```python
from build123d import *

# Parameters (mm, degrees)
SKETCH019_R          = 1.7
PAD002_DEPTH         = 13
SKETCH020_W          = 7
SKETCH020_H          = 8
POCKET017_DEPTH      = 7
POCKET019_DEPTH      = 8
POCKET020_DEPTH      = 8
SKETCH024_R          = 2.5
SKETCH025_R          = 10
SKETCH027_R          = 10
SKETCH026_R          = 2.5
SKETCH021_R          = 1.7
POCKET021_DEPTH      = 21.5010001
POCKET021_DEPTH_BACK = 21.5010001
SKETCH028_W          = 57.890867
SKETCH028_H          = 28.005435
SKETCH028_W_2        = 40
SKETCH028_H_2        = 13
POCKET022_DEPTH      = 21.5010001
POCKET022_DEPTH_BACK = 21.5010001
SKETCH029_W          = 10.751613
SKETCH029_H          = 15.361299
POCKET023_DEPTH      = 5
SKETCH030_W          = 5.428132
SKETCH030_H          = 4.529939
POCKET024_DEPTH      = 5


with BuildPart() as part:
    # Sketch019 → Pad002 (new body)
    with BuildSketch(Plane.XY):
        Polygon((-13.5, -16), (13.5, -16), (13.5, 6), (13.5, 24), (-13.5, 24), (-13.5, 6), align=None)
        with Locations((10, 10)):
            Circle(SKETCH019_R, mode=Mode.SUBTRACT)
        with Locations((-10, 10)):
            Circle(SKETCH019_R, mode=Mode.SUBTRACT)
        with Locations((-10, -10)):
            Circle(SKETCH019_R, mode=Mode.SUBTRACT)
        with Locations((10, -10)):
            Circle(SKETCH019_R, mode=Mode.SUBTRACT)
    extrude(amount=PAD002_DEPTH)

    # Sketch020 → Pocket017 (cut)
    with BuildSketch(Plane.XY.offset(13)):
        Polygon((-2.25, -8), (4.75, -8), (4.75, -16), (13.5, -16), (13.5, -6), (-0.5, -6), (-0.5, 1), (8, 1), (8, 24), (-8, 24), (-8, 6), (-13.5, 6), (-13.5, -16), (-2.25, -16), align=None)
        with Locations((1.25, 7)):
            Rectangle(SKETCH020_W, SKETCH020_H, mode=Mode.SUBTRACT)
    extrude(amount=-POCKET017_DEPTH, mode=Mode.SUBTRACT)

    # Sketch022 → Pocket019 (cut)
    with BuildSketch(Plane.YZ.offset(4)):
        Polygon((19.6, 6.5), (17.8, 9.6176914536), (14.2, 9.6176914536), (12.4, 6.5), (14.2, 3.3823085464), (17.8, 3.3823085464), align=None)
    extrude(amount=POCKET019_DEPTH, mode=Mode.SUBTRACT)

    # Sketch023 → Pocket020 (cut)
    with BuildSketch(Plane.YZ.offset(-4)):
        Polygon((19.6, 6.5), (17.8, 9.6176914536), (14.2, 9.6176914536), (12.4, 6.5), (14.2, 3.3823085464), (17.8, 3.3823085464), align=None)
    extrude(amount=-POCKET020_DEPTH, mode=Mode.SUBTRACT)

    # Sketch024 → AdditiveLoft section 0
    with BuildSketch(Plane.YZ.offset(21.5)):
        with Locations((16, 6.5)):
            Circle(SKETCH024_R)
    # Sketch025 → AdditiveLoft section 1
    with BuildSketch(Plane.YZ.offset(13.5)):
        with Locations((16, 6.5)):
            Circle(SKETCH025_R)
    loft()

    # Sketch027 → AdditiveLoft001 section 0
    with BuildSketch(Plane.YZ.offset(-13.5)):
        with Locations((16, 6.5)):
            Circle(SKETCH027_R)
    # Sketch026 → AdditiveLoft001 section 1
    with BuildSketch(Plane.YZ.offset(-21.5)):
        with Locations((16, 6.5)):
            Circle(SKETCH026_R)
    loft()

    # Sketch021 → Pocket021 (cut, two sides)
    with BuildSketch(Plane.YZ) as pocket021_sk:
        with Locations((16, 6.5)):
            Circle(SKETCH021_R)
    extrude(amount=-POCKET021_DEPTH, mode=Mode.SUBTRACT)
    extrude(pocket021_sk.sketch, amount=POCKET021_DEPTH_BACK, mode=Mode.SUBTRACT)

    # Sketch028 → Pocket022 (cut, two sides)
    with BuildSketch(Plane.YZ) as pocket022_sk:
        with Locations((4.9093215, 6.8553455)):
            Rectangle(SKETCH028_W, SKETCH028_H)
        with Locations((4, 6.5)):
            Rectangle(SKETCH028_W_2, SKETCH028_H_2, mode=Mode.SUBTRACT)
    extrude(amount=-POCKET022_DEPTH, mode=Mode.SUBTRACT)
    extrude(pocket022_sk.sketch, amount=POCKET022_DEPTH_BACK, mode=Mode.SUBTRACT)

    # Sketch029 (on DatumPlane) → Pocket023 (cut)
    with BuildSketch(Plane(origin=(11.8478062442, -4.3122488143, 9.8505836052), x_dir=(0.5785325453, -0.210568626, -0.7880107536), z_dir=(0.7404878903, -0.2695155509, 0.6156614753))):
        with Locations((-0.9861515, 3.6505885)):
            Rectangle(SKETCH029_W, SKETCH029_H)
    extrude(amount=POCKET023_DEPTH, mode=Mode.SUBTRACT)

    # Sketch030 (on DatumPlane) → Pocket024 (cut)
    with BuildSketch(Plane(origin=(0, 0, 25), x_dir=(0.2777686245, 0.2484410627, 0.9279663947), z_dir=(-0.6924826787, -0.6177293717, 0.3726636058))):
        with Locations((-14.088813, 13.6448355)):
            Rectangle(SKETCH030_W, SKETCH030_H)
    extrude(amount=POCKET024_DEPTH, mode=Mode.SUBTRACT)


solid = part.part
```
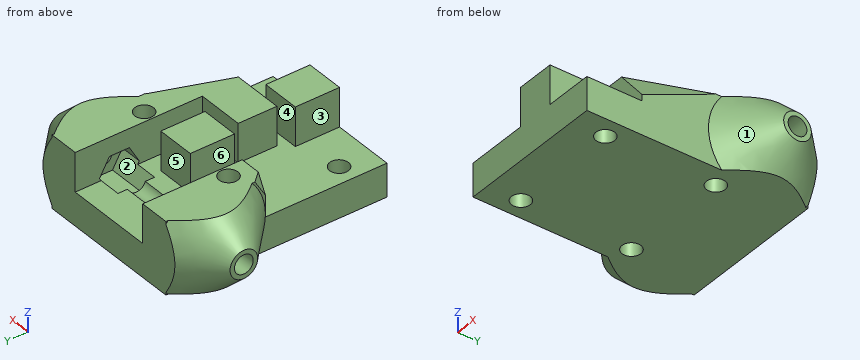
Here's how the part is built. I have some questions about the finished solid (model axes, mm). Face numbers are marked on the shaded views. A direction names the side the tool comes from. Give positions to 0.01 mm unless a question says otherwise; leave off trailing zeros. Order: outer loops, then holes, each group sorted by start corner. A loop starts at its lowest first (then second) coordinate and runs counter-clockwise, first axis right, second up. Notation, with made-up numbers: (62, 17) -> (87, 17) arc R24 ccw to (87, 55) -> close; hole circle Ø3 at (-37.75, 85.25). An arc over 180 degrees is marked (long way). Use CSV: the item, a comma, the result in double quotes. Start each with the question number.
Item 1: Suppose I cut it at C-C (y = -13). List the corners of the cut face in (x, z) for me, and give its area (3 significant figures).
Item 2: Suppose I cut it at A-A (x = -10). List the corners of the cut face in (y, z) for me, and give its area (3 significant figures).
Item 3: Suppose I cut it at D-D (x = 1.5). List the corners of the cut face in (y, z) for me.
Item 4: If I drill on probe 1 along X at (y, z) = (-10, 4.7); probe 2 along Y at (x, z) = (10, 3.25); probe 3 along X at (y, z) = (9, 11.5), over which ranges is the centre line in solid material (lowest first)? Write a range as [from, to].
Item 5: On a 3-axis mill with a long thin cutter (end or side, diameter ignored), from which of +Z, -Z, +X, -X, +Y, -Y can I reach the whole of each face in a straight line? I mean the marked faces 4, 5 and 6. Say none if no direction works.
Item 6: Suppose I cut it at B-B (y = 16). List the corners of the cut face in (x, z) for me.
Item 7: Thinking about a two-plate mould opening in Y: for the marked faces 1, 2 and 3, which applies, pulls with the +Y half, pulls with the -Y half, needs draft (parallel to the pull), parting line crosses it, or undercut?
Item 8: I'm going to push flat-ended pins straight in: P1, Ø2, axis at y = -10.5, z = 9.5, coming from the -X side; P2, Ø4.5, axis at x = 10, y = -10, coming from the +Z side; P3, Ø3, axis at y = 15, z = 6, coming from the +X side; P4, Ø4, axis at y = 0.5, z = 4.5, coming from the +X side. Where does each tip first touch, or does it pass through?
Answer block:
1,outline,"(-13.5, 0) -> (13.5, 0) -> (13.5, 6) -> (4.75, 6) -> (4.75, 13) -> (-2.25, 13) -> (-2.25, 6) -> (-13.5, 6) -> close"
1,area,"211 mm^2"
2,outline,"(-16, 0) -> (-11.7, 0) -> (-11.7, 6) -> (-16, 6) -> close; (-8.3, 0) -> (8.3, 0) -> (8.3, 13) -> (6, 13) -> (6, 6) -> (-8.3, 6) -> close; (11.7, 0) -> (24, 0) -> (24, 13) -> (11.7, 13) -> close; hole (12.4, 6.5) -> (14.2, 3.38) -> (17.8, 3.38) -> (19.6, 6.5) -> (17.8, 9.62) -> (14.2, 9.62) -> close"
2,area,"268 mm^2"
3,outline,"(-16, 0) -> (24, 0) -> (24, 6) -> (17.62, 6) arc R1.7 cw to (14.38, 6) -> (11, 6) -> (11, 13) -> (3, 13) -> (3, 6) -> (1, 6) -> (1, 13) -> (-6, 13) -> (-6, 6) -> (-8, 6) -> (-8, 13) -> (-16, 13) -> close"
4,probe 1,"x = [-13.5, -11.7], [-8.3, 8.3], [11.7, 13.5]"
4,probe 2,"y = [-16, -11.7], [-8.3, 8.3], [11.7, 24]"
4,probe 3,"x = [-14.99, -11.37], [-8.63, -8], [-2.25, 4.75], [8, 8.63], [11.37, 14.99]"
5,face 4,"+Z, +X, -X"
5,face 5,"+Z, +Y"
5,face 6,"+Z, +Y, -Y"
6,outline,"(-21.5, 4) -> (-17.23, 0) -> (17.23, 0) -> (21.5, 4) -> (21.5, 4.8) -> (12, 4.8) -> (12, 3.38) -> (4, 3.38) -> (4, 4.8) -> (-4, 4.8) -> (-4, 3.38) -> (-12, 3.38) -> (-12, 4.8) -> (-21.5, 4.8) -> close; (-21.5, 8.2) -> (-12, 8.2) -> (-12, 9.62) -> (-8, 9.62) -> (-8, 13) -> (-17.23, 13) -> (-21.5, 9) -> close; (8, 9.62) -> (12, 9.62) -> (12, 8.2) -> (21.5, 8.2) -> (21.5, 9) -> (17.23, 13) -> (8, 13) -> close"
7,face 1,"parting line crosses it"
7,face 2,"undercut"
7,face 3,"needs draft"
8,P1,"stops at x = -2.25"
8,P2,"stops at z = 6"
8,P3,"stops at x = 21.5"
8,P4,"stops at x = 13.5"
